Check sheet for the modelled part. Datum: model origin and axes. Units: mm. A direction names the side the tool comes from. Round coordinates to 2 decimals unless told otherwise and drop trailing zeros. Loops run counter-clockwise (first coordinate to the right, second up) from the corner with the lowest first, then second, coordinate; pieces in that order, holes last. Notation, with made-up numbers: (30.25, -33.5) -> (81.25, -33.5) arc R11 cw to (81.25, -26.5) -> close; hole circle Ø10 at (-2.75, 85). An arc over 180 degrees is marked (long way). One line per item, written item: value. Start each with the question number.
1. Release check for a two-part mould opening along X. For faces 1 (the face through (50.8, 0, 6)), 2 (the face through (12.114, 3.815, 6.261)), 3 (the face through (8, 12, 0)) record: +X half, -X half, draft (parallel to the pull), parting line (faces both ways), or undercut.
2. Set-up check for faces 4 (the face through (17.274, -0.356, 9.989)), 5 (the face through (44.361, 1.707, 9.027)), 6 (the face through (35, 0, 12.7)), 7 (the face through (0, -18, 10.922)): record each of +Z, -Z, +X, -X, +Y, -Y from which the full face is reachable in a straight line by a thin tool's end or side.
3. Cross-section at D-D on y = -18. Record the cut outline in (x, z).
4. Cross-section at B-B on z = 6.35. Record the cut outline in (x, y) (3 decimals), then the cut area to 3 significant figures.
5. Go/stop test with flat-tipped pins: pin 1 (5 mm diameter, centred on x = 0.5, y = -20, fed in from +Z); pin 2 (0.5 mm diameter, centred on y = -21, z = 12, fed in from +X). Record where each tip stops, or that it passes through.
6. Cross-section at C-C on x = 0. Record the cut outline in (y, z).
7. Cross-section at A-A on y = 0. Record the cut outline in (x, z) (3 decimals), then the cut area to 3 significant figures.
8. Material ranges on L1, parallel to X at y = 0, z = 5.5; L2, parallel to Y at x = 0, z = 8; L3, parallel to X at y = 0, z = 8.75, recorded low to high.
from build123d import *

# Parameters (mm, degrees)
F0_W     = 76.2
F0_H     = 50.8
F0_R     = 12.7
F1_DEPTH = 12.7
F3_DEPTH = 1.778
F5_DEPTH = 50.8
F6_R     = 3.175
F7_DEPTH = 12.7


with BuildPart() as f1:
    # F0 (on Top) → F1 (new body)
    with BuildSketch(Plane.XY):
        Rectangle(F0_W, F0_H)
        Circle(F0_R, mode=Mode.SUBTRACT)
    extrude(amount=F1_DEPTH)

    # F2 (on face) → F3 (cut)
    with BuildSketch(Plane.XY.offset(12.7)):
        with BuildLine():
            Line((4.8691992944, 25.4), (-5.2908007056, 25.4))
            Line((-5.2908007056, 25.4), (-5.2908007056, 11.545450528))
            ThreePointArc((-5.2908007056, 11.545450528), (-0.2300096138, 12.6979169779), (4.8691992944, 11.7294884045))
            Line((4.8691992944, 11.7294884045), (4.8691992944, 25.4))
        make_face()
        with BuildLine():
            Line((-5.2908007056, -11.545450528), (-5.2908007056, -25.4))
            Line((-5.2908007056, -25.4), (4.8691992944, -25.4))
            Line((4.8691992944, -25.4), (4.8691992944, -11.7294884045))
            ThreePointArc((4.8691992944, -11.7294884045), (-0.2300096138, -12.6979169779), (-5.2908007056, -11.545450528))
        make_face()
        with BuildLine():
            Line((-5.2908007056, 11.545450528), (-5.2908007056, -11.545450528))
            ThreePointArc((-5.2908007056, -11.545450528), (-0.2300096138, -12.6979169779), (4.8691992944, -11.7294884045))
            Line((4.8691992944, -11.7294884045), (4.8691992944, 11.7294884045))
            ThreePointArc((4.8691992944, 11.7294884045), (-0.2300096138, 12.6979169779), (-5.2908007056, 11.545450528))
        make_face()
    extrude(amount=-F3_DEPTH, mode=Mode.SUBTRACT)

    # F4 (on face) → F5 (cut, through all)
    with BuildSketch(Plane.XZ.offset(25.4)):
        Polygon((31.5391992944, 12.7), (18.8391992944, 12.7), (15.6641992944, 7.200738686), (34.7141992944, 7.200738686), align=None)
    extrude(amount=-F5_DEPTH, mode=Mode.SUBTRACT)

    # F6 (on face) → F7 (join)
    with BuildSketch(Plane.YZ.offset(38.1)):
        with Locations((0, 6.35)):
            Circle(F6_R)
    extrude(amount=F7_DEPTH)


solid = f1.part
Taken from the geometry:
1. face 1: +X half
1. face 2: undercut
1. face 3: draft
2. face 4: +Y, -Y
2. face 5: +X
2. face 6: +Z, +X, -X, +Y, -Y
2. face 7: +Z, +Y, -Y
3. outline: (-38.1, 0) -> (38.1, 0) -> (38.1, 12.7) -> (31.54, 12.7) -> (34.71, 7.2) -> (15.66, 7.2) -> (18.84, 12.7) -> (4.87, 12.7) -> (4.87, 10.92) -> (-5.29, 10.92) -> (-5.29, 12.7) -> (-38.1, 12.7) -> close
4. outline: (-38.1, -25.4) -> (38.1, -25.4) -> (38.1, -3.175) -> (50.8, -3.175) -> (50.8, 3.175) -> (38.1, 3.175) -> (38.1, 25.4) -> (-38.1, 25.4) -> close; hole circle Ø25.4 at (0, 0)
4. area: 3,440 mm2
5. pin 1: stops at z = 10.92
5. pin 2: stops at x = 38.1
6. outline: (-25.4, 0) -> (-12.7, 0) -> (-12.7, 10.92) -> (-25.4, 10.92) -> close; (12.7, 0) -> (25.4, 0) -> (25.4, 10.92) -> (12.7, 10.92) -> close
7. outline: (-38.1, 0) -> (-12.7, 0) -> (-12.7, 12.7) -> (-38.1, 12.7) -> close; (12.7, 0) -> (38.1, 0) -> (38.1, 3.175) -> (50.8, 3.175) -> (50.8, 9.525) -> (38.1, 9.525) -> (38.1, 12.7) -> (31.539, 12.7) -> (34.714, 7.201) -> (15.664, 7.201) -> (18.839, 12.7) -> (12.7, 12.7) -> close
7. area: 639 mm2
8. L1: x = -38.1 to -12.7, 12.7 to 50.8
8. L2: y = -25.4 to -12.7, 12.7 to 25.4
8. L3: x = -38.1 to -12.7, 12.7 to 16.56, 33.82 to 50.8
